from build123d import *

# Parameters (mm, degrees)
EXTRUDE_1_DEPTH     = 40
EXTRUDE_2_DEPTH     = 12
SKETCH_3_W          = 9.8
SKETCH_3_H          = 45.5
CUT_EXTRUDE_1_DEPTH = 10
SKETCH_4_W          = 9.8
SKETCH_4_H          = 48.5
CUT_EXTRUDE_2_DEPTH = 5.5
SKETCH_5_R          = 1.1
CUT_EXTRUDE_3_DEPTH = 56.154328933
SKETCH_6_W          = 3.5
SKETCH_6_H          = 35
CUT_EXTRUDE_4_DEPTH = 55.525223521
SKETCH_7_R          = 1.1
CUT_EXTRUDE_5_DEPTH = 55.525223521
SKETCH_8_R          = 1.95
CUT_EXTRUDE_6_DEPTH = 1.2
FILLET_2_R          = 1


with BuildPart() as part:
    # 草图1 → 凸台-拉伸1 (new body)
    with BuildSketch(Plane(origin=(0, 0, 0), x_dir=(1, 0, 0), z_dir=(0, 1, 0))):
        Polygon((-6, 11.5), (-7.763269807, 1.5), (7.763269807, 1.5), (6, 11.5), align=None)
        Polygon((-7.763269807, 1.5), (-8.292250749, -1.5), (8.292250749, -1.5), (7.763269807, 1.5), align=None)
        Polygon((-13, 1.5), (-13, -1.5), (-8.292250749, -1.5), (-7.763269807, 1.5), align=None)
        Polygon((7.763269807, 1.5), (8.292250749, -1.5), (13, -1.5), (13, 1.5), align=None)
    extrude(amount=EXTRUDE_1_DEPTH)

    # 草图2 → 凸台-拉伸2 (add)
    with BuildSketch(Plane(origin=(0, 40, 0), x_dir=(1, 0, 0), z_dir=(0, 1, 0))):
        Polygon((6, 11.5), (7.763269807, 1.5), (7.763269807, -1.5), (-7.763269807, -1.5), (-7.763269807, 1.5), (-6, 11.5), align=None)
    extrude(amount=EXTRUDE_2_DEPTH)

    # 草图3 → 切除-拉伸1 (cut)
    with BuildSketch(Plane.XY.offset(1.5)):
        with Locations((0, 25.75)):
            Rectangle(SKETCH_3_W, SKETCH_3_H)
    extrude(amount=-CUT_EXTRUDE_1_DEPTH, mode=Mode.SUBTRACT)

    # 草图4 → 切除-拉伸2 (cut)
    with BuildSketch(Plane.XY.offset(1.5)):
        with Locations((0, 25.75)):
            Rectangle(SKETCH_4_W, SKETCH_4_H)
    extrude(amount=-CUT_EXTRUDE_2_DEPTH, mode=Mode.SUBTRACT)

    # 草图5 → 切除-拉伸3 (cut, through all)
    with BuildSketch(Plane.XY.offset(1.5)):
        with Locations((-10.5, 36)):
            Circle(SKETCH_5_R)
        with Locations(Location((-10.5, 4, 0), (0, 0, 180))):
            Circle(SKETCH_5_R)
        with Locations((10.5, 4)):
            Circle(SKETCH_5_R)
        with Locations(Location((10.5, 36, 0), (0, 0, 180))):
            Circle(SKETCH_5_R)
    extrude(amount=-CUT_EXTRUDE_3_DEPTH, mode=Mode.SUBTRACT)

    # 草图6 → 切除-拉伸4 (cut, through all)
    with BuildSketch(Plane.XY.offset(-8.5)):
        with Locations((0, 25.75)):
            Rectangle(SKETCH_6_W, SKETCH_6_H)
    extrude(amount=-CUT_EXTRUDE_4_DEPTH, mode=Mode.SUBTRACT)

    # 草图7 → 切除-拉伸5 (cut, through all)
    with BuildSketch(Plane.XY.offset(-8.5)):
        with Locations((0, 46.25)):
            Circle(SKETCH_7_R)
        with Locations(Location((0, 5.25, 0), (0, 0, 180))):
            Circle(SKETCH_7_R)
    extrude(amount=-CUT_EXTRUDE_5_DEPTH, mode=Mode.SUBTRACT)

    # 草图8 → 切除-拉伸6 (cut)
    with BuildSketch(Plane(origin=(0, 0, -11.5), x_dir=(-1, 0, 0), z_dir=(0, 0, -1))):
        with Locations((0, 46.25)):
            Circle(SKETCH_8_R)
        with Locations((0, 5.25)):
            Circle(SKETCH_8_R)
    extrude(amount=-CUT_EXTRUDE_6_DEPTH, mode=Mode.SUBTRACT)

    # 圆角2
    fillet_2_edges = [part.edges().sort_by_distance(p)[0] for p in [
        (6, 26, -11.5),
        (-6, 26, -11.5),
    ]]
    fillet(fillet_2_edges, radius=FILLET_2_R)


solid = part.part
CAD build for the part. Positions are in the model's coordinates, mm. A direction names the side the tool comes from. Coordinates: 2 decimals unless noted, no trailing zeros. Write each loop counter-clockwise with the first axis right and the second up, starting at its lowest first coordinate (ties: lowest second). Pieces come first, ordered by that corner, then holes. Notation, with made-up numbers: M 82.5,23 L 104.5,23 A21 ccw 104.5,33 Z; hole C 65,9 d9. An arc over 180 degrees is marked long. Answer as a JSON object with one key per item and string values. Group by question number.
1) Saw through at D-D (z = -7.5). Write the cut outline in (x, y), plus the area to 3 significant figures.
2) Pin check, flat tips, straight feed: pin 1 Ø2 at (x, y) = (0, 5.25) entering from +Z; pin 2 Ø1.5 at (x, z) = (0.5, -9.5) entering from -Y; pin 3 Ø1.5 at (x, z) = (-11.5, -0.5) entering from +Y; pin 4 Ø1.2 at (x, y) = (2, 49) entering from +Z. Stop position of each tip, or through.
3) Saw through at C-C (x = 0). Give the number of separate pieces and of enclosed holes in the cut face, plus the area to 3 significant figures.
4) Saw through at A-A (y = 22). Write the cut outline in (x, z).
5) Saw through at B-B (x = -10.5). Write the cut outline in (y, z), plus the area to 3 significant figures.
6) Mould opens along X. For faces 5 (the face through (9.91, 35.07, 0.02)), 6 (the face through (0.59, 47.18, -9.39)), 7 (the face through (5.81, 26.36, -11.26)), 8 (the face through (0, 0, -4)) say: +X half, -X half, draft (parallel to the pull), parting line (faces both ways), or undercut.
7) Tool access for faces 1 (the face through (4.9, 25, -3)), 2 (the face through (10, 20, -1.5)), 3 (the face through (1.75, 26, -10)), 4 (the face through (0.423, 44.346, -10.908)): list every direction of +Z, -Z, +X, -X, +Y, -Y with a clear straight run to the whole face (end or side of a thin tool).
8) Wall check: line 1 (Y direction, x = -10.5, z = 0.85); line 2 (Y direction, x = 0, z = -9.05); line 3 (Y direction, x = 0, z = -10.65). Give the ranges that are in metal, low to high. Write a range as from..to.
Values follow:
{
 "1": {"outline": "M -6.71,0 L 6.71,0 L 6.71,52 L -6.71,52 Z; hole M -4.9,3 L 4.9,3 L 4.9,48.5 L -4.9,48.5 Z", "area": "251 mm2"},
 "2": {"pin 1": "passes through", "pin 2": "stops at y = 0", "pin 3": "stops at y = 40", "pin 4": "stops at z = -4"},
 "3": {"separate pieces": "4", "enclosed holes": "0", "area": "82.2 mm2"},
 "4": {"outline": "M -13,-1.5 L -7.76,-1.5 L -6.15,-10.67 A1 ccw -5.16,-11.5 L -1.75,-11.5 L -1.75,-8.5 L -4.9,-8.5 L -4.9,1.5 L -13,1.5 Z; M 1.75,-11.5 L 5.16,-11.5 A1 ccw 6.15,-10.67 L 7.76,-1.5 L 13,-1.5 L 13,1.5 L 4.9,1.5 L 4.9,-8.5 L 1.75,-8.5 Z"},
 "5": {"outline": "M 0,-1.5 L 2.9,-1.5 L 2.9,1.5 L 0,1.5 Z; M 5.1,-1.5 L 34.9,-1.5 L 34.9,1.5 L 5.1,1.5 Z; M 37.1,-1.5 L 40,-1.5 L 40,1.5 L 37.1,1.5 Z", "area": "107 mm2"},
 "6": {"face 5": "undercut", "face 6": "undercut", "face 7": "+X half", "face 8": "draft"},
 "7": {"face 1": "+Z", "face 2": "-Z, +X, +Y, -Y", "face 3": "+Z, -Z", "face 4": "-Z"},
 "8": {"line 1": "y = 0..2.9, 5.1..34.9, 37.1..40", "line 2": "y = 0..4.15, 6.35..8.25, 43.25..45.15, 47.35..52", "line 3": "y = 0..3.3, 7.2..8.25, 43.25..44.3, 48.2..52"}
}
